For this review, take the finished solid that the model builds, in its own axes (mm). A direction names the side the tool comes from. Round coordinates to 2 decimals unless told otherwise and drop trailing zeros. Write each loop counter-clockwise with the first axis right and the second up, starting at its lowest first coordinate (ties: lowest second). Pieces come first, ordered by that corner, then holes. Notation, with made-up numbers: (-18.75, 67) - (-6.75, 67) arc R13 ccw to (-6.75, 73) - close; hole circle Ø10 at (17, 2). An arc over 180 degrees is marked (long way). One line per item, written item: value. Start each with the question number.
Q1. Add section A-A on x = -65. Write out the cut boundary in (y, z).
Q2. Add section C-C on y = -0.8. Write out the cut boundary in (x, z), and give its area (3 significant figures).
Q3. Add section D-D on z = -73. Write out the cut boundary in (x, y), and give its area (4 significant figures).
Q4. Add section B-B on z = 44. Write out the cut boundary in (x, y).
Q5. Clearance check with a flat-ended pin moving along its axis: pin 1 Ø3 at (x, z) = (-43.5, 66) entering from +Y. State where the tip first meets the part, or that it passes through.
Q6. Mouldability with a two-part tool opening along X and no side actions: class faces 3 (the face through (133.342, -0.493, 94.904)), 4 (the face through (104.74, -0.49, -55.85)), 5 (the face through (-132.869, -0.493, 95.596)), 6 (the face through (-2, -1, 2)) as +X half, -X half, draft (parallel to the pull), parting line (faces both ways), or undercut.
Q7. For probe 1 along Z at (x, y) = (-65, -0.65); probe 2 along Z at (x, y) = (69.5, -0.55); probe 3 along X at (y, z) = (-0.55, -55.5), list the stretches that pass through material, from the lowest coordinate up.
Q8. Tool access review of faces 1 (the face through (-2, 0, 2)), 2 (the face through (9.26, -0.49, -90.15)): name each direction out of +Z, -Z, +X, -X, +Y, -Y from which nothing blocks a thin tool from reaching the whole face with its end or side.
```python
from build123d import *

# Parameters (mm, degrees)
F0_R     = 11
F0_R_2   = 21.5
F1_DEPTH = 1


with BuildPart() as f1:
    # F0 (on Front) → F1 (new body)
    with BuildSketch(Plane.XZ):
        Polygon((-150, -120), (150, -120), (150, 70.5), (116.211094, 120), (-116.211094, 120), (-150, 70.5), align=None)
        with Locations((-65, -73)):
            Circle(F0_R, mode=Mode.SUBTRACT)
        with BuildLine():
            ThreePointArc((107.75, -83), (104.821068, -90.071068), (97.75, -93))
            Line((97.75, -93), (16.25, -93))
            ThreePointArc((16.25, -93), (9.178932, -90.071068), (6.25, -83))
            Line((6.25, -83), (6.25, -63))
            ThreePointArc((6.25, -63), (9.178932, -55.928932), (16.25, -53))
            Line((16.25, -53), (97.75, -53))
            ThreePointArc((97.75, -53), (104.821068, -55.928932), (107.75, -63))
            Line((107.75, -63), (107.75, -83))
        make_face(mode=Mode.SUBTRACT)
        with Locations((-65, 44)):
            Circle(F0_R_2, mode=Mode.SUBTRACT)
    extrude(amount=F1_DEPTH)


solid = f1.part
```
Result set:
1. outline: (-1, -120) - (0, -120) - (0, -84) - (-1, -84) - close; (-1, -62) - (0, -62) - (0, 22.5) - (-1, 22.5) - close; (-1, 65.5) - (0, 65.5) - (0, 120) - (-1, 120) - close
2. outline: (-150, -120) - (150, -120) - (150, 70.5) - (116.21, 120) - (-116.21, 120) - (-150, 70.5) - close; hole circle Ø43 at (-65, 44); hole circle Ø22 at (-65, -73); hole (6.25, -83) arc R10 ccw to (16.25, -93) - (97.75, -93) arc R10 ccw to (107.75, -83) - (107.75, -63) arc R10 ccw to (97.75, -53) - (16.25, -53) arc R10 ccw to (6.25, -63) - close
2. area: 64,500 mm^2
3. outline: (-150, -1) - (-76, -1) - (-76, 0) - (-150, 0) - close; (-54, -1) - (6.25, -1) - (6.25, 0) - (-54, 0) - close; (107.75, -1) - (150, -1) - (150, 0) - (107.75, 0) - close
3. area: 176.5 mm^2
4. outline: (-150, -1) - (-86.5, -1) - (-86.5, 0) - (-150, 0) - close; (-43.5, -1) - (150, -1) - (150, 0) - (-43.5, 0) - close
5. pin 1: stops at y = 0
6. face 3: +X half
6. face 4: undercut
6. face 5: -X half
6. face 6: draft
7. probe 1: z = -120 to -84, -62 to 22.5, 65.5 to 120
7. probe 2: z = -120 to -93, -53 to 120
7. probe 3: x = -150 to 9.64, 104.36 to 150
8. face 1: +Z, -Z, +X, -X, +Y
8. face 2: +Y, -Y
